Read the model definition and answer for the solid it produces. Units are mm, in the model's axes. Coordinates: 2 decimals unless noted, no trailing zeros. Loops run counter-clockwise (first coordinate to the right, second up) from the corner with the lowest first, then second, coordinate; pieces in that order, holes last.
from build123d import *

# Parameters (mm, degrees)
CUT_EXTRUDE1_DEPTH = 30
CUT_EXTRUDE2_DEPTH = 30


with BuildPart() as part:
    # Sketch1 → Revolve1 (revolve)
    with BuildSketch(Plane(origin=(0, 0, 0), x_dir=(1, 0, 0), z_dir=(0, 1, 0))):
        with BuildLine():
            Line((-3, -15), (-3, 15))
            ThreePointArc((-3, 15), (-3.645751311, 19.291502622), (0, 21.645751311))
            Line((0, 21.645751311), (0, 20.345751311))
            ThreePointArc((0, 20.345751311), (-2.7, 17.645751311), (0, 14.945751311))
            Line((0, 14.945751311), (0, 13.645751311))
            Line((0, 13.645751311), (0, -13.645751311))
            Line((0, -13.645751311), (0, -14.945751311))
            ThreePointArc((0, -14.945751311), (-2.7, -17.645751311), (0, -20.345751311))
            Line((0, -20.345751311), (0, -21.645751311))
            ThreePointArc((0, -21.645751311), (-3.645751311, -19.291502622), (-3, -15))
        make_face()
    revolve(axis=Axis((0, 0, -91.394122854), (0, 0, 1)))

    # Sketch2 → Cut-Extrude1 (cut, symmetric)
    with BuildSketch(Plane(origin=(0, 0, 0), x_dir=(1, 0, 0), z_dir=(0, 1, 0))):
        with BuildLine():
            Line((-1.2, 15.107825257), (-1.2, 1.596713369))
            ThreePointArc((-1.2, 1.596713369), (-0.907106781, 0.889606588), (-0.2, 0.596713369))
            Line((-0.2, 0.596713369), (0.2, 0.596713369))
            ThreePointArc((0.2, 0.596713369), (0.907106781, 0.889606588), (1.2, 1.596713369))
            Line((1.2, 1.596713369), (1.2, 15.107825257))
            ThreePointArc((1.2, 15.107825257), (1.284324545, 15.509743733), (1.523076923, 15.843879024))
            ThreePointArc((1.523076923, 15.843879024), (0, 19.75), (-1.523076923, 15.843879024))
            ThreePointArc((-1.523076923, 15.843879024), (-1.284324545, 15.509743733), (-1.2, 15.107825257))
        make_face()
        with BuildLine():
            Line((-1.2, -15.107825257), (-1.2, -1.596713369))
            ThreePointArc((-1.2, -1.596713369), (-0.907106781, -0.889606588), (-0.2, -0.596713369))
            Line((-0.2, -0.596713369), (0.2, -0.596713369))
            ThreePointArc((0.2, -0.596713369), (0.907106781, -0.889606588), (1.2, -1.596713369))
            Line((1.2, -1.596713369), (1.2, -15.107825257))
            ThreePointArc((1.2, -15.107825257), (1.284324545, -15.509743733), (1.523076923, -15.843879024))
            ThreePointArc((1.523076923, -15.843879024), (0, -19.75), (-1.523076923, -15.843879024))
            ThreePointArc((-1.523076923, -15.843879024), (-1.284324545, -15.509743733), (-1.2, -15.107825257))
        make_face()
    extrude(amount=CUT_EXTRUDE1_DEPTH, both=True, mode=Mode.SUBTRACT)

    # Sketch3 → Cut-Extrude2 (cut, symmetric)
    with BuildSketch(Plane(origin=(0, 0, 0), x_dir=(0, 0, -1), z_dir=(1, 0, 0))):
        Polygon((0, -2), (70.025003907, -2), (70.025003907, -4), (-79.974996093, -4), (-79.974996093, -2), align=None)
        Polygon((0, 2), (70.025003907, 2), (70.025003907, 4), (-79.974996093, 4), (-79.974996093, 2), align=None)
    extrude(amount=CUT_EXTRUDE2_DEPTH, both=True, mode=Mode.SUBTRACT)


solid = part.part
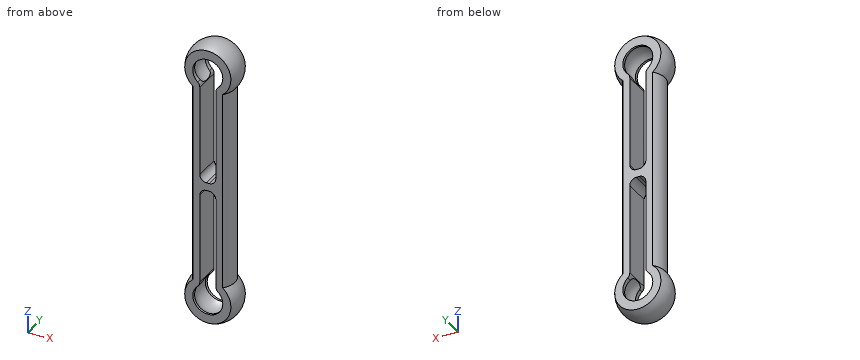
Item 1: Find the intervals of material crossed by line 1 along Z through (x, y) = (2, -1.15); line 2 along Z through (x, y) = (0, -1.75); line 3 along X through (y, z) = (1.5, 17.5), in increasing order.
Numbers:
line 1: z = -20.91 to -19.05, -16.24 to 16.24, 19.05 to 20.91
line 2: z = -21.24 to -19.75, -0.6 to 0.6, 19.75 to 21.24
line 3: x = -3.71 to -2.25, 2.25 to 3.71
Item 2: A cutting plane is placed at D-D on z = 1. Determine the outline of the cut face in (x, y), then the cut area to 3 significant figures.
Numbers:
outline: (-2.24, -2) - (-1, -2) - (-1, 2) - (-2.24, 2) arc R3 ccw to start; (1, -2) - (2.24, -2) arc R3 ccw to (2.24, 2) - (1, 2) - close
area: 14.1 mm2
Item 3: A cutting plane is placed at A-A on z = 8.5. Determine the outline of the cut face in (x, y), then the cut area to 3 significant figures.
Numbers:
outline: (-2.24, -2) - (-1.2, -2) - (-1.2, 2) - (-2.24, 2) arc R3 ccw to start; (1.2, -2) - (2.24, -2) arc R3 ccw to (2.24, 2) - (1.2, 2) - close
area: 12.5 mm2
Item 4: A cutting plane is placed at B-B on y = -0.8. Determine the outline of the cut face in (x, z).
Numbers:
outline: (-2.89, -15) arc R3.92 ccw (long way) to (2.89, -15) - (2.89, 15) arc R3.92 ccw (long way) to (-2.89, 15) - close; hole (-1.24, -15.38) arc R2.58 ccw (long way) to (1.24, -15.38) arc R1 cw to (1.2, -15.11) - (1.2, -1.6) arc R1 ccw to (0.2, -0.6) - (-0.2, -0.6) arc R1 ccw to (-1.2, -1.6) - (-1.2, -15.11) arc R1 cw to start; hole (-1.24, 15.38) arc R1 cw to (-1.2, 15.11) - (-1.2, 1.6) arc R1 ccw to (-0.2, 0.6) - (0.2, 0.6) arc R1 ccw to (1.2, 1.6) - (1.2, 15.11) arc R1 cw to (1.24, 15.38) arc R2.58 ccw (long way) to start
Item 5: Given pin 1 (2 mm diameter, centred on x = 0, y = 1.5, fed in from -Z); pin 2 (2 mm diameter, centred on x = -1.5, y = -1, fed in from +Z); pin 3 (1.5 mm diameter, centred on y = 1, z = 10.5, fed in from -X), each flat-ended and moving along its own axis, determine where each tip first touches the part or whether it passes through.
Numbers:
pin 1: stops at z = -21.61
pin 2: stops at z = 21.56
pin 3: stops at x = -2.99
Item 6: A cutting plane is placed at C-C on z = 17.5. Determine the outline of the cut face in (x, y), then the cut area to 3 significant figures.
Numbers:
outline: (-3.46, -2) - (-2.25, -2) - (-2.25, -1.49) arc R2.7 cw to (-2.25, 1.49) - (-2.25, 2) - (-3.46, 2) arc R4 ccw to start; (2.25, -2) - (3.46, -2) arc R4 ccw to (3.46, 2) - (2.25, 2) - (2.25, 1.49) arc R2.7 cw to (2.25, -1.49) - close
area: 10.8 mm2
